Job drawing, mm, ordinate dimensions from the low corner. One solid piece. Give positions to 0.01 mm unless a question says otherwise; leave off trailing zeros. Order: outer loops, then holes, each group sorted by start corner. A loop starts at its lowest first (then second) coordinate and runs counter-clockwise, first axis right, second up. Notation, with made-up numbers: (7, 57) - (45, 57) arc R16 ccw to (45, 72) - close; hole circle Ø3 at (67, 65.5). An arc over 180 degrees is marked (long way). One line per item, written item: value.
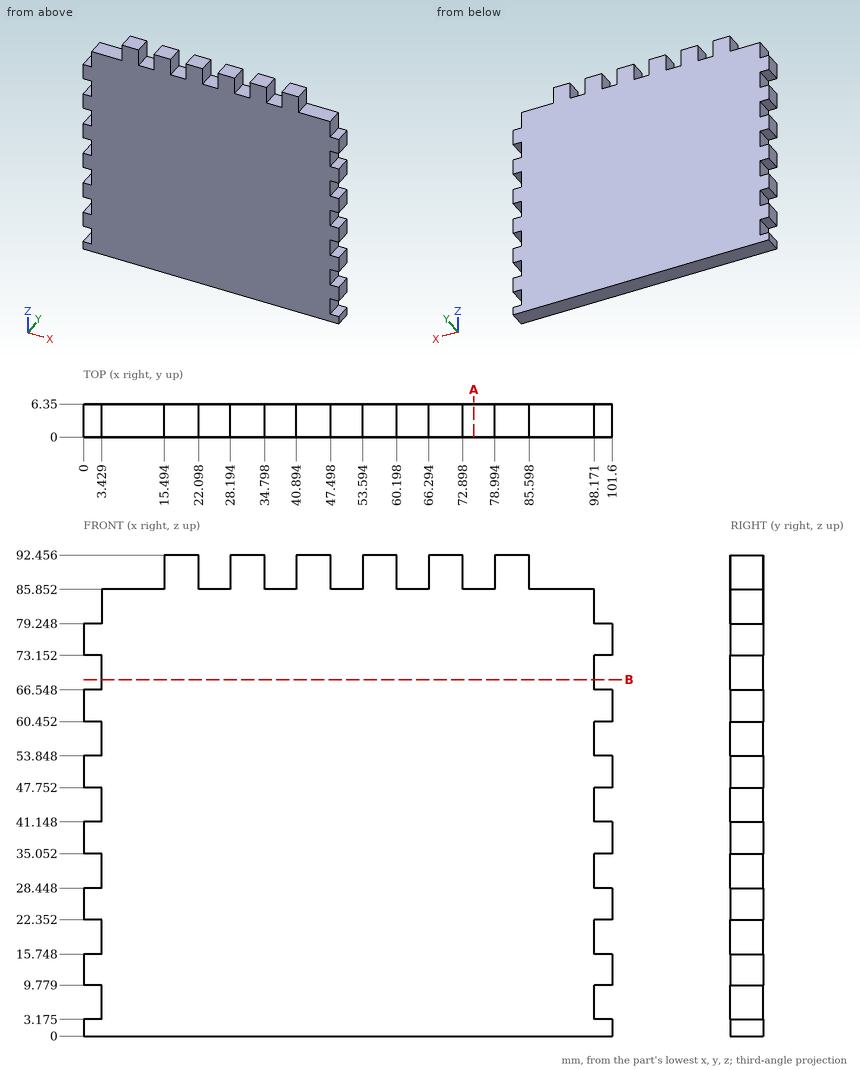
1) Slice it at A-A on x = 75. Write the cut outline in (y, z).
Answer:
outline: (0, 0) - (6.35, 0) - (6.35, 85.85) - (0, 85.85) - close
2) Wall check: line 1 along X through (y, z) = (2.25, 47); line 2 along Z through (x, y) = (28, 3.5). Give the ranges that are in metal, low to high. Write a range as [from, to].
Answer:
line 1: x = [3.43, 98.17]
line 2: z = [0, 85.85]
3) Drop flat-ended pins along their axis: P1, Ø2.5, axis at x = 2.5, y = 2, coming from the +Z side; P2, Ø3, axis at y = 2, z = 90, coming from the -X side; P3, Ø3, axis at y = 2.5, z = 70, coming from the +X side. Give the stop position or say it passes through.
Answer:
P1: stops at z = 85.85
P2: stops at x = 15.49
P3: stops at x = 98.17
4) Slice it at B-B on z = 68.5. Write the cut outline in (x, y), then the cut area to 3 significant figures.
Answer:
outline: (3.43, 0) - (98.17, 0) - (98.17, 6.35) - (3.43, 6.35) - close
area: 602 mm2
